Can you work these out from the model? Positions are in its coordinate system, mm. A direction names the side the tool comes from. Round coordinates to 2 decimals unless told otherwise and drop trailing zeros. Loops run counter-clockwise (first coordinate to the right, second up) from the corner with the lowest first, then second, coordinate; pieces in that order, holes last. Notation, with made-up numbers: M 68.25,-14 L 101.25,-14 A22 cw 101.25,-7 Z; hole C 31.5,40.25 d2. An arc over 180 degrees is marked long. Return JSON: item names as keys, results as strings.
```python
from build123d import *

# Parameters (mm, degrees)
SKETCH1_W               = 152.4
SKETCH1_H               = 50.8
BOSS_EXTRUDE1_DEPTH     = 3.175
SKETCH2_W               = 12.7
SKETCH2_H               = 14.2875
CUT_EXTRUDE1_DEPTH      = 4.175
SKETCH3_R               = 0.79375
CUT_EXTRUDE2_DEPTH      = 4.175
F_1_4_CLEARANCE_HOLE1_D = 6.7564
F_10_CLEARANCE_HOLE1_D  = 5.1054


with BuildPart() as part:
    # Sketch1 → Boss-Extrude1 (new body)
    with BuildSketch(Plane.XY):
        with Locations((76.2, 25.4)):
            Rectangle(SKETCH1_W, SKETCH1_H)
    extrude(amount=BOSS_EXTRUDE1_DEPTH)

    # Sketch2 → Cut-Extrude1 (cut, through all)
    with BuildSketch(Plane.XY.offset(3.175)):
        with Locations((6.35, 43.65625)):
            Rectangle(SKETCH2_W, SKETCH2_H)
        with Locations((6.35, 7.14375)):
            Rectangle(SKETCH2_W, SKETCH2_H)
        with Locations((146.05, 7.14375)):
            Rectangle(SKETCH2_W, SKETCH2_H)
        with Locations((146.05, 43.65625)):
            Rectangle(SKETCH2_W, SKETCH2_H)
    extrude(amount=-CUT_EXTRUDE1_DEPTH, mode=Mode.SUBTRACT)

    # Sketch3 → Cut-Extrude2 (cut, through all)
    with BuildSketch(Plane.XY.offset(3.175)):
        with Locations((12.7, 37.30625)):
            Circle(SKETCH3_R)
        with Locations((12.7, 13.49375)):
            Circle(SKETCH3_R)
        with Locations((139.7, 13.49375)):
            Circle(SKETCH3_R)
        with Locations((139.7, 37.30625)):
            Circle(SKETCH3_R)
    extrude(amount=-CUT_EXTRUDE2_DEPTH, mode=Mode.SUBTRACT)

    # 1/4 Clearance Hole1 (through all)
    with Locations(Plane.XY.offset(3.175)):
        with Locations((6.35, 25.4), (146.05, 25.4)):
            Hole(F_1_4_CLEARANCE_HOLE1_D / 2)

    # #10 Clearance Hole1 (through all)
    with Locations(Plane.XY.offset(3.175)):
        with Locations((76.2, 4.7625), (90.7, 4.7625), (61.7, 4.7625), (61.7, 46.0375), (76.2, 46.0375), (90.7, 46.0375)):
            Hole(F_10_CLEARANCE_HOLE1_D / 2)


solid = part.part
```
Q1. If I drill on line 1 along Y through (x, z) = (76.2, 2.4); line 2 along Y through (x, z) = (139.5, 2.05); line 3 along X through (y, z) = (44, 1.05), over which ranges is the centre line in solid material (lowest first)?
Results:
{"line 1": "y = 0 to 2.21, 7.32 to 43.48, 48.59 to 50.8", "line 2": "y = 0 to 12.73, 14.26 to 36.54, 38.07 to 50.8", "line 3": "x = 12.7 to 60.16, 63.24 to 74.66, 77.74 to 89.16, 92.24 to 139.7"}
Q2. Suppose I cut it at A-A, the plane x = 146.05. Please give me the cut outline in (y, z) (1 decimal), plus the area to 3 significant figures.
Results:
{"outline": "M 14.3,0 L 22,0 L 22,3.2 L 14.3,3.2 Z; M 28.8,0 L 36.5,0 L 36.5,3.2 L 28.8,3.2 Z", "area": "49.1 mm2"}
Q3. On a 3-axis mill with a long thin cutter (end or side, diameter ignored), from which of +Z, -Z, +X, -X, +Y, -Y can I reach the whole of each face in a straight line? I mean faces 1 (the flat face through (6, 14.288, 2)), 2 (the flat face through (12.7, 44, 2)), 3 (the flat face through (146, 14.288, 2)), 4 (the flat face through (146, 36.512, 2)), 5 (the cylindrical face through (78.75, 4.87, 1.57)). Say none if no direction works.
Results:
{"face 1": "+Z, -Z, -X, -Y", "face 2": "+Z, -Z, -X, +Y", "face 3": "+Z, -Z, +X, -Y", "face 4": "+Z, -Z, +X, +Y", "face 5": "+Z, -Z"}
Q4. I'm going to push flat-ended pins straight in: pin 1 Ø4 at (x, y) = (57.5, 44.5) entering from -Z; pin 2 Ø4 at (x, y) = (76.2, 46.04) entering from +Z; pin 3 Ø1 at (x, z) = (6.5, 1.5) entering from +Y. Where does each tip first touch, or does it pass through?
Results:
{"pin 1": "stops at z = 0", "pin 2": "passes through", "pin 3": "stops at y = 36.51"}
Q5. Thinking about a two-plate mould opening in X: for faces 6 (the flat face through (75, 50.8, 2)), 7 (the cylindrical face through (88.265, 5.529, 1.565)), 8 (the flat face through (0, 25, 2)), 9 (the flat face through (139.7, 44, 2)), which applies, pulls with the +X half, pulls with the -X half, needs draft (parallel to the pull), parting line crosses it, or undercut?
Results:
{"face 6": "needs draft", "face 7": "undercut", "face 8": "pulls with the -X half", "face 9": "pulls with the +X half"}
Q6. Suppose I cut it at B-B, the plane y = 25.4. Please give me the cut outline in (x, z) (3 decimals).
Results:
{"outline": "M 0,0 L 2.972,0 L 2.972,3.175 L 0,3.175 Z; M 9.728,0 L 142.672,0 L 142.672,3.175 L 9.728,3.175 Z; M 149.428,0 L 152.4,0 L 152.4,3.175 L 149.428,3.175 Z"}
Q7. Suppose I cut it at D-D, the plane z = 0.7. State how many separate pieces and enclosed holes the cut face has, plus the area to 3 significant figures.
Results:
{"separate pieces": "1", "enclosed holes": "8", "area": "6,820 mm2"}
Q8. Suppose I cut it at C-C, the plane x = 76.2. Please give me the cut outline in (y, z) (3 decimals).
Results:
{"outline": "M 0,0 L 2.21,0 L 2.21,3.175 L 0,3.175 Z; M 7.315,0 L 43.485,0 L 43.485,3.175 L 7.315,3.175 Z; M 48.59,0 L 50.8,0 L 50.8,3.175 L 48.59,3.175 Z"}
